Could you check a few things on this model? Use its own coordinates, in mm. A direction names the side the tool comes from. Give positions to 0.01 mm unless a question says otherwise; leave off trailing zeros. Loops run counter-clockwise (first coordinate to the right, second up) from the corner with the lowest first, then second, coordinate; pieces in that order, holes last. Notation, with made-up numbers: M -11.5,12.5 L 36.5,12.5 A23 cw 36.5,50.5 Z; hole C 33,89 d1. An arc over 180 degrees is marked long. Answer in a Markdown table with one row per item. Add a question column.
1. Which directions (+Z, -Z, +X, -X, +Y, -Y) give clear straight access to the entire face, cutting with the end or side of a thin tool? Please do faces 4 (the flat face through (41777.543, -386, 8)), 5 (the cylindrical face through (41771.522, -385.608, -21.647)).
2. Thinking about a two-plate mould opening in Z: for faces 1 (the flat face through (41771, -386, 32.353)), 2 (the cylindrical face through (41771.46, -385.61, -53.85)), 3 (the flat face through (41772, -384.087, 1)), which applies, released by +Z, released by -Z, zero draft, split by the parting line, or undercut?
3. If we section it at C-C on z = 36: List the corners of the cut face in (x, y) for me, then the cut area to 3 significant figures.
4. If we section it at A-A on z = -18: List the corners of the cut face in (x, y) for me.
5. If we section it at D-D on z = 11: List the corners of the cut face in (x, y) for me.
6. I need wall thicknesses on line 1 along X through (y, z) = (-385.9, 35.5); line 2 along X through (y, z) = (-386.1, -14); line 3 along X through (y, z) = (-385.7, -17.5). Which ranges of each line are inside material? Lowest first, please. Write a range as from..to.
7. I'm going to push flat-ended pins straight in: pin 1 Ø0.7 at (y, z) = (-385.5, -49.5) entering from +X; pin 2 Ø1.5 at (y, z) = (-386, 28) entering from -X; pin 3 Ø0.9 at (y, z) = (-385, 10) entering from +X. Where does each tip first touch, or does it pass through?
8. If we section it at B-B on y = -385: Count the separate pieces of the cut face and the enclosed holes in it, then the cut area to 3 significant figures.
```python
from build123d import *

# Parameters (mm, degrees)
CROQUIS1_R                 = 1.5
CROQUIS1_R_2               = 3.75
CROQUIS1_W                 = 3
CROQUIS1_H                 = 6
CROQUIS1_H_2               = 9
SALIENTE_EXTRUIR1_DEPTH    = 3
S_LIDO_MOVER_COPIAR1_ANGLE = 90


with BuildPart() as part:
    # Croquis1 → Saliente-Extruir1 (new body)
    with BuildSketch(Plane.XY):
        with BuildLine():
            Line((41777.543498403, -351.025953533), (41777.543498403, -434.939495491))
            ThreePointArc((41777.543498403, -434.939495491), (41771.543498403, -440.939495491), (41765.543498403, -434.939495491))
            Line((41765.543498403, -434.939495491), (41765.543498403, -351.025953694))
            ThreePointArc((41765.543498403, -351.025953694), (41763.543498332, -345.734451045), (41765.543498332, -340.44294837))
            ThreePointArc((41765.543498332, -340.44294837), (41767.026813105, -337.979872872), (41767.543498332, -335.151445748))
            Line((41767.543498332, -335.151445748), (41767.543498332, -334.234450911))
            ThreePointArc((41767.543498332, -334.234450911), (41771.543498261, -330.234450982), (41775.54349819, -334.234450911))
            Line((41775.54349819, -334.234450911), (41775.54349819, -335.151445587))
            ThreePointArc((41775.54349819, -335.151445587), (41776.060183455, -337.979872812), (41777.543498332, -340.44294837))
            ThreePointArc((41777.543498332, -340.44294837), (41779.543498332, -345.734450938), (41777.543498403, -351.025953533))
        make_face()
        with Locations((41771.543498403, -434.939495491)):
            Circle(CROQUIS1_R, mode=Mode.SUBTRACT)
        with Locations((41771.543498545, -389.939495491)):
            Circle(CROQUIS1_R, mode=Mode.SUBTRACT)
        with Locations((41771.543498332, -345.734450992)):
            Circle(CROQUIS1_R_2, mode=Mode.SUBTRACT)
        with BuildLine():
            Line((41772.543498261, -333.234450911), (41772.543498261, -337.234450911))
            ThreePointArc((41772.543498261, -337.234450911), (41771.543498261, -338.234450911), (41770.543498261, -337.234450911))
            Line((41770.543498261, -337.234450911), (41770.543498261, -333.234450911))
            ThreePointArc((41770.543498261, -333.234450911), (41771.543498261, -332.234450911), (41772.543498261, -333.234450911))
        make_face(mode=Mode.SUBTRACT)
        with BuildLine():
            Line((41772.543498545, -363.439495491), (41772.543498545, -368.439495491))
            ThreePointArc((41772.543498545, -368.439495491), (41771.543498545, -369.439495491), (41770.543498545, -368.439495491))
            Line((41770.543498545, -368.439495491), (41770.543498545, -363.439495491))
            ThreePointArc((41770.543498545, -363.439495491), (41771.543498545, -362.439495491), (41772.543498545, -363.439495491))
        make_face(mode=Mode.SUBTRACT)
        with Locations((41771.043498545, -379.439495491)):
            Rectangle(CROQUIS1_W, CROQUIS1_H, mode=Mode.SUBTRACT)
        with Locations((41771.043498545, -420.939495491)):
            Rectangle(CROQUIS1_W, CROQUIS1_H_2, mode=Mode.SUBTRACT)
    extrude(amount=SALIENTE_EXTRUIR1_DEPTH)


with BuildPart() as part_1:
    # Sólido-Mover/Copiar1: moved
    add(part.part.rotate(Axis((0, -385.586973236, 1.5), (-1, 0, 0)), S_LIDO_MOVER_COPIAR1_ANGLE))


solid = part_1.part
```
Results:
| question | item | result |
|---|---|---|
| 1 | face 4 | +Z, +X, +Y, -Y |
| 1 | face 5 | +Y, -Y |
| 2 | face 1 | undercut |
| 2 | face 2 | released by -Z |
| 2 | face 3 | zero draft |
| 3 | outline | M 41765.54,-387.09 L 41769.54,-387.09 L 41769.54,-384.09 L 41765.54,-384.09 Z; M 41772.54,-387.09 L 41777.54,-387.09 L 41777.54,-384.09 L 41772.54,-384.09 Z |
| 3 | area | 27.0 mm2 |
| 4 | outline | M 41765.54,-387.09 L 41770.54,-387.09 L 41770.54,-384.09 L 41765.54,-384.09 Z; M 41772.54,-387.09 L 41777.54,-387.09 L 41777.54,-384.09 L 41772.54,-384.09 Z |
| 5 | outline | M 41765.54,-387.09 L 41777.54,-387.09 L 41777.54,-384.09 L 41765.54,-384.09 Z |
| 6 | line 1 | 41765.54..41769.54, 41772.54..41777.54 |
| 6 | line 2 | 41765.54..41777.54 |
| 6 | line 3 | 41765.54..41770.54, 41772.54..41777.54 |
| 7 | pin 1 | x = 41775.54 |
| 7 | pin 2 | x = 41765.54 |
| 7 | pin 3 | x = 41777.54 |
| 8 | separate pieces | 1 |
| 8 | enclosed holes | 7 |
| 8 | area | 1,170 mm2 |
